The listing builds one solid part. Answer for the finished solid, in the listing's coordinates (mm). A direction names the side the tool comes from. Round coordinates to 2 decimals unless told otherwise and drop trailing zeros. Write each loop counter-clockwise with the first axis right and the second up, starting at its lowest first coordinate (ties: lowest second). Pieces come first, ordered by that corner, then holes. Notation, with made-up numbers: (73, 67.25) - (103, 67.25) arc R19 cw to (103, 72.25) - close; hole circle Ø8 at (-15.5, 38). An arc over 180 degrees is marked (long way). Answer in a Markdown table with one row per item.
from build123d import *

# Parameters (mm, degrees)
F0_W     = 39.610392
F0_H     = 50
F0_R     = 2.49857
F1_DEPTH = 10


with BuildPart() as f1:
    # F0 (on Top) → F1 (new body)
    with BuildSketch(Plane.XY):
        with Locations((0, 2.218615)):
            Rectangle(F0_W, F0_H)
        with BuildLine():
            ThreePointArc((17.439984, -9.515637), (0.515297, -16.475749), (-16.40939, -9.515637))
            add(Edge.make_bspline(
                [(0, -13.069506), (-2.759309, -17.431528), (-11.705375, -13.140691), (-16.40939, -9.515637)],
                knots=[0, 0, 0, 0, 16.789821, 16.789821, 16.789821, 16.789821], degree=3))
            add(Edge.make_bspline(
                [(0, -13.069506), (2.521035, -17.431528), (13.085214, -12.930726), (17.439984, -9.515637)],
                knots=[0, 0, 0, 0, 17.7984, 17.7984, 17.7984, 17.7984], degree=3))
        make_face(mode=Mode.SUBTRACT)
        with Locations((-15.692642, 22.781385)):
            Circle(F0_R, mode=Mode.SUBTRACT)
        with BuildLine():
            Line((-6.628194, 3.720442), (0, 23.035537))
            Line((0, 23.035537), (6.628194, 3.720442))
            ThreePointArc((6.628194, 3.720442), (10.016927, 0.025924), (15.030141, 0))
            ThreePointArc((15.030141, 0), (13.392417, -2.906154), (13.481836, -6.240802))
            add(Edge.make_bspline(
                [(13.481836, -6.240802), (9.220885, -5.342014), (6.425123, -11.953733), (2.150824, -12.901068)],
                knots=[0, 0, 0, 0, 13.143476, 13.143476, 13.143476, 13.143476], degree=3))
            add(Edge.make_bspline(
                [(2.150824, -12.901068), (11.792642, -9.865808), (0.927339, 8.11935), (0, 18.521211)],
                knots=[0, 0, 0, 0, 31.495803, 31.495803, 31.495803, 31.495803], degree=3))
            add(Edge.make_bspline(
                [(-2.150824, -12.901068), (-11.827089, -9.865808), (-0.506544, 8.11935), (0, 18.521211)],
                knots=[0, 0, 0, 0, 31.495803, 31.495803, 31.495803, 31.495803], degree=3))
            add(Edge.make_bspline(
                [(-13.481836, -6.240802), (-9.247256, -5.342014), (-6.102542, -11.953733), (-2.150824, -12.901068)],
                knots=[0, 0, 0, 0, 13.143476, 13.143476, 13.143476, 13.143476], degree=3))
            ThreePointArc((-13.481836, -6.240802), (-13.392417, -2.906154), (-15.030141, 0))
            ThreePointArc((-15.030141, 0), (-10.016927, 0.025924), (-6.628194, 3.720442))
        make_face(mode=Mode.SUBTRACT)
    extrude(amount=F1_DEPTH)


solid = f1.part
(1) For a pull along X with two mould halves and no side action, classify faces 3 (the cylindrical face through (-13.38, -2.95, 4.93)), 4 (the flat face through (19.805, 2, 5)), 5 (the flat face through (0, 3, 0)) as pulls with the +X half, pulls with the -X half, needs draft (parallel to the pull), parting line crosses it, or undercut.
Checked values:
| item | result |
|---|---|
| face 3 | undercut |
| face 4 | pulls with the +X half |
| face 5 | needs draft |
(2) Section A-A (x = -17) is taken. Give the vertices of the cut face in (y, z), and give its area (3 significant figures).
Checked values:
| item | result |
|---|---|
| outline | (-22.78, 0) - (20.65, 0) - (20.65, 10) - (-22.78, 10) - close; (24.91, 0) - (27.22, 0) - (27.22, 10) - (24.91, 10) - close |
| area | 457 mm2 |
(3) For faces 1 (the flat face through (-19.805, 2, 5)), 2 (the flat face through (3.27, 13.51, 4.93)), determine the directions among +Z, -Z, +X, -X, +Y, -Y from which every point of the face is accessible in a straight line to the end or side of a thin tool.
Checked values:
| item | result |
|---|---|
| face 1 | +Z, -Z, -X, +Y, -Y |
| face 2 | +Z, -Z |
(4) A flat-ended cylindrical pin translates along its axis: pin 1 (6.5 mm diameter, centred on x = -15.69, y = 22.78, fed in from +Z). Find the tip coordinate at first contact, or state that the pin passes through.
Checked values:
| item | result |
|---|---|
| pin 1 | stops at z = 10 |
(5) Find the intervals of material crossed by line 1 (X direction, y = 21, z = 2.5); line 2 (X direction, y = 2, z = 7.5); line 3 (Y direction, x = 7.5, z = 2.75), in increasing order.
Checked values:
| item | result |
|---|---|
| line 1 | x = -19.81 to -17.44, -13.94 to -0.7, 0.7 to 19.81 |
| line 2 | x = -19.81 to -7.54, -4.33 to 4.49, 7.54 to 19.81 |
| line 3 | y = -22.78 to -15.44, -14.35 to -9.18, 2.05 to 27.22 |
(6) Section B-B (y = 2) is taken. State how many separate pieces and enclosed holes the cut face has, and give its area (3 significant figures).
Checked values:
| item | result |
|---|---|
| separate pieces | 3 |
| enclosed holes | 0 |
| area | 334 mm2 |
